Geometry: final body of the model. Coordinates: model frame, mm. A direction names the side the tool comes from. Give positions to 0.01 mm unless a question says otherwise; leave off trailing zeros. Loops run counter-clockwise (first coordinate to the right, second up) from the corner with the lowest first, then second, coordinate; pieces in that order, holes last.
```python
from build123d import *

# Parameters (mm, degrees)
SKETCH_1_R      = 1.6
EXTRUDE_1_DEPTH = 3


with BuildPart() as part:
    # 草图1 → 凸台-拉伸1 (new body)
    with BuildSketch(Plane(origin=(0, 0, 0), x_dir=(1, 0, 0), z_dir=(0, 1, 0))):
        with BuildLine():
            Line((-25.423831263, 10.512307079), (44.076168737, 10.512307079))
            Line((44.076168737, 10.512307079), (44.076168737, 22.012307079))
            Line((44.076168737, 22.012307079), (47.076168737, 22.012307079))
            Line((47.076168737, 22.012307079), (47.076168737, 15.012307079))
            Line((47.076168737, 15.012307079), (52.490895584, 15.012307079))
            Line((52.490895584, 15.012307079), (52.490895584, 38.012307079))
            Line((52.490895584, 38.012307079), (47.076168737, 38.012307079))
            Line((47.076168737, 38.012307079), (47.076168737, 31.012307079))
            Line((47.076168737, 31.012307079), (44.076168737, 31.012307079))
            Line((44.076168737, 31.012307079), (44.076168737, 80.512307079))
            Line((44.076168737, 80.512307079), (47.076168737, 80.512307079))
            Line((47.076168737, 80.512307079), (47.076168737, 73.512307079))
            Line((47.076168737, 73.512307079), (52.490895584, 73.512307079))
            Line((52.490895584, 73.512307079), (52.490895584, 96.512307079))
            Line((52.490895584, 96.512307079), (47.076168737, 96.512307079))
            Line((47.076168737, 96.512307079), (47.076168737, 89.512307079))
            Line((47.076168737, 89.512307079), (44.076168737, 89.512307079))
            Line((44.076168737, 89.512307079), (44.076168737, 96.512307079))
            Line((44.076168737, 96.512307079), (20.576168737, 96.512307079))
            Line((20.576168737, 96.512307079), (20.576168737, 76.566499541))
            ThreePointArc((20.576168737, 76.566499541), (20.284948115, 76.523300877), (19.990895584, 76.508854947))
            Line((19.990895584, 76.508854947), (9.576168737, 76.508854947))
            ThreePointArc((9.576168737, 76.508854947), (7.454848394, 77.387534604), (6.576168737, 79.508854947))
            Line((6.576168737, 79.508854947), (6.576168737, 83.508854947))
            ThreePointArc((6.576168737, 83.508854947), (9.576168737, 86.508854947), (12.576168737, 83.508854947))
            Line((12.576168737, 83.508854947), (12.576168737, 79.508854947))
            Line((12.576168737, 79.508854947), (14.576168737, 79.508854947))
            Line((14.576168737, 79.508854947), (14.576168737, 96.512307079))
            Line((14.576168737, 96.512307079), (-25.423831263, 96.512307079))
            Line((-25.423831263, 96.512307079), (-25.423831263, 89.512307079))
            Line((-25.423831263, 89.512307079), (-28.423831263, 89.512307079))
            Line((-28.423831263, 89.512307079), (-28.423831263, 96.512307079))
            Line((-28.423831263, 96.512307079), (-33.838558109, 96.512307079))
            Line((-33.838558109, 96.512307079), (-33.838558109, 73.512307079))
            Line((-33.838558109, 73.512307079), (-28.423831263, 73.512307079))
            Line((-28.423831263, 73.512307079), (-28.423831263, 80.512307079))
            Line((-28.423831263, 80.512307079), (-25.423831263, 80.512307079))
            Line((-25.423831263, 80.512307079), (-25.423831263, 31.012307079))
            Line((-25.423831263, 31.012307079), (-28.423831263, 31.012307079))
            Line((-28.423831263, 31.012307079), (-28.423831263, 38.012307079))
            Line((-28.423831263, 38.012307079), (-33.838558109, 38.012307079))
            Line((-33.838558109, 38.012307079), (-33.838558109, 15.012307079))
            Line((-33.838558109, 15.012307079), (-28.423831263, 15.012307079))
            Line((-28.423831263, 15.012307079), (-28.423831263, 22.012307079))
            Line((-28.423831263, 22.012307079), (-25.423831263, 22.012307079))
            Line((-25.423831263, 22.012307079), (-25.423831263, 10.512307079))
        make_face()
        with Locations(Location((-10.423831263, 29.512307079, 0), (0, 0, 270))):
            Circle(SKETCH_1_R, mode=Mode.SUBTRACT)
        with Locations(Location((18.576168737, 29.512307079, 0), (0, 0, 270))):
            Circle(SKETCH_1_R, mode=Mode.SUBTRACT)
        with Locations(Location((18.576168737, 61.512307079, 0), (0, 0, 270))):
            Circle(SKETCH_1_R, mode=Mode.SUBTRACT)
        with Locations(Location((-10.423831263, 61.512307079, 0), (0, 0, 270))):
            Circle(SKETCH_1_R, mode=Mode.SUBTRACT)
        with Locations(Location((-26.923831263, 26.512307079, 0), (0, 0, 270))):
            Circle(SKETCH_1_R, mode=Mode.SUBTRACT)
        with Locations(Location((45.576168737, 26.512307079, 0), (0, 0, 270))):
            Circle(SKETCH_1_R, mode=Mode.SUBTRACT)
        with Locations(Location((45.576168737, 85.012307079, 0), (0, 0, 270))):
            Circle(SKETCH_1_R, mode=Mode.SUBTRACT)
        with Locations(Location((-26.923831263, 85.012307079, 0), (0, 0, 270))):
            Circle(SKETCH_1_R, mode=Mode.SUBTRACT)
    extrude(amount=EXTRUDE_1_DEPTH)


solid = part.part
```
Q1. Pin query (flat end, axial travel): pin 1 Ø1 at (y, z) = (0.5, -45) entering from +X; pin 2 Ø1.9 at (x, z) = (-26.92, -26.51) entering from +Y; pin 3 Ø1.5 at (x, y) = (-27, 1.5) entering from -Z; pin 4 Ø1 at (y, z) = (1, -62) entering from -X. Return the tip coordinate at first contact, or that it passes through.
Q2. Material intervals for probe 1 along X at (y, z) = (1.5, -75); probe 2 along X at (y, z) = (2.8, -90.5); probe 3 along Z at (x, y) = (48.5, 2.8), sorted ascending.
Q3. Section query B-B, the plane z = -85.5. Return loops of the section in (x, y).
Q4. Section query D-D, the plane z = -64.5. Return loops of the section in (x, y), and give its area (4 significant figures).
Q5. Mould query, pull axis Z, two halves, no side actions, for faces 1 (the face through (-27, 1, -89.512)), 2 (the face through (-25.424, 1, -93)), 3 (the face through (12.576, 1, -82)). Classes: +Z half, -Z half, draft (parallel to the pull), parting line (faces both ways), or undercut.
Q6. Section query A-A, the plane z = -74.5. Return loops of the section in (x, y).
Q7. Reachability of faces 4 (the face through (44.076, 1, -93)), 5 (the face through (47.076, 1, -77)), 6 (the face through (-31, 1, -15.012)) from +Z, -Z, +X, -X, +Y, -Y: full face, straight path, thin tool, end or side. Return the list, or none.
Q8. Section query C-C, the plane y = 0.85. State how many separate pieces and enclosed holes the cut face has, and give its area (3 significant figures).
Resolved:
1. pin 1: stops at x = 44.08
1. pin 2: passes through
1. pin 3: stops at z = -89.51
1. pin 4: stops at x = -25.42
2. probe 1: x = -33.84 to -28.42, -25.42 to 44.08, 47.08 to 52.49
2. probe 2: x = -33.84 to -28.42, -25.42 to 14.58, 20.58 to 44.08, 47.08 to 52.49
2. probe 3: z = -96.51 to -73.51, -38.01 to -15.01
3. outline: (-33.84, 0) - (-28.45, 0) - (-28.45, 3) - (-33.84, 3) - close; (-25.4, 0) - (7.33, 0) - (7.33, 3) - (-25.4, 3) - close; (11.82, 0) - (14.58, 0) - (14.58, 3) - (11.82, 3) - close; (20.58, 0) - (44.05, 0) - (44.05, 3) - (20.58, 3) - close; (47.1, 0) - (52.49, 0) - (52.49, 3) - (47.1, 3) - close
4. outline: (-25.42, 0) - (44.08, 0) - (44.08, 3) - (-25.42, 3) - close
4. area: 208.5 mm2
5. face 1: -Z half
5. face 2: draft
5. face 3: undercut
6. outline: (-33.84, 0) - (-28.42, 0) - (-28.42, 3) - (-33.84, 3) - close; (-25.42, 0) - (44.08, 0) - (44.08, 3) - (-25.42, 3) - close; (47.08, 0) - (52.49, 0) - (52.49, 3) - (47.08, 3) - close
7. face 4: -Z, +Y, -Y
7. face 5: +Y, -Y
7. face 6: +Z, -X, +Y, -Y
8. separate pieces: 1
8. enclosed holes: 8
8. area: 6,340 mm2
